Design review of the part built by this model. Coordinates are the model's own, in mm. A direction names the side the tool comes from. Coordinates: 2 decimals unless noted, no trailing zeros. Loops run counter-clockwise (first coordinate to the right, second up) from the corner with the lowest first, then second, coordinate; pieces in that order, holes last. Notation, with made-up numbers: M -39.75,-20 L 11.25,-20 A28 ccw 11.25,8 Z; hole C -21,-18 d10. An arc over 180 degrees is marked long. Answer as CSV lines item,"result". Start each with the question number.
from build123d import *

# Parameters (mm, degrees)
PAD002_DEPTH    = 7
SKETCH025_R     = 3
POCKET018_DEPTH = 15
POCKET019_DEPTH = 98.908358
SKETCH028_R     = 3
POCKET021_DEPTH = 7.001


with BuildPart() as part:
    # Sketch023 → Pad002 (new body)
    with BuildSketch(Plane.XY):
        with BuildLine():
            Line((75.261973, 88.907358), (50.261973, 88.907358))
            Line((50.261973, 84.907358), (50.261973, 88.907358))
            Line((50.261973, 84.907358), (20.261973, 84.907358))
            Line((-9.396926, 3.420201), (20.261973, 84.907358))
            ThreePointArc((-9.396926, 3.420201), (-4.942745, -8.693059), (7.744606, -6.326221))
            Line((7.744606, -6.326221), (52.028155, 47.886022))
            ThreePointArc((75.261973, 58.907358), (62.404289, 56.012339), (52.028155, 47.886022))
            Line((75.261973, 88.907358), (75.261973, 58.907358))
        make_face()
    extrude(amount=PAD002_DEPTH)

    # Sketch025 (on Face4 of Pad002) → Pocket018 (cut)
    with BuildSketch(Plane(origin=(0, 84.907358, 0), x_dir=(-1, 0, 0), z_dir=(0, 1, 0))):
        with Locations((-35.261973, 3.5)):
            Circle(SKETCH025_R)
    extrude(amount=-POCKET018_DEPTH, mode=Mode.SUBTRACT)

    # Sketch026 (on Face2 of Pocket018) → Pocket019 (cut, through all)
    with BuildSketch(Plane(origin=(0, 88.907358, 0), x_dir=(-1, 0, 0), z_dir=(0, 1, 0))):
        Polygon((-75.261973, 7), (-75.261973, 0), (-71.220521, 7), align=None)
    extrude(amount=-POCKET019_DEPTH, mode=Mode.SUBTRACT)

    # Sketch028 → Pocket021 (cut, through all)
    with BuildSketch(Plane.XY.offset(7)):
        with Locations((54.303425, 73.770624)):
            Circle(SKETCH028_R)
    extrude(amount=-POCKET021_DEPTH, mode=Mode.SUBTRACT)


with BuildPart() as part_1:
    # Body002 placement: moved
    add(part.part.moved(Location((-250, 0, 0))))


with BuildPart() as part_2:
    # Clone placement: moved
    add(part_1.part.moved(Location((262, 76, 0))))


solid = part_2.part
Item 1: Mouldability with a two-part tool opening along Z and no side actions: class faces 1 (the face through (50.26, 153.51, 3.63)), 2 (the face through (47.5, 160.907, 0.3)), 3 (the face through (85.27, 149.98, 3.45)) as released by +Z, released by -Z, zero draft, split by the parting line, or undercut.
Item 2: For pin 1 (2 mm diameter, centred on x = 40.5, z = 4, fed in from +Y); pin 2 (1.5 mm diameter, centred on x = 21, z = 2, fed in from -Y); pin 3 (1.8 mm diameter, centred on x = 46, z = 5, fed in from +Y), all flat-tipped, find the tip position at first contact; note any pin that passes through.
Item 3: Add section C-C (y = 99). Give the boundary of the cut face in (x, z).
Item 4: Add section A-A (z = 3.5). Give the boundary of the cut face in (x, y).
Item 5: For faces 4 (the face through (62.262, 163, 3)), 5 (the face through (47, 145.907, 4)), 6 (the face through (65.913, 152.745, 3.549)), list the 3-axis set-ups (+Z, -Z, +X, -X, +Y, -Y) from which the entire face can be reached by the end or side of a thin tool; tool diameter is ignored.
Item 6: For line 1 along Y through (x, z) = (69, 2); line 2 along X through (y, z) = (110, 5.25); line 3 along Y through (x, z) = (34.5, 1), list the stretches that pass through material, from the lowest coordinate up. Write a range as from..to.
Item 7: Add section B-B (x = 13.5). Give the boundary of the cut face in (y, z), plus the area to 3 significant figures.
Response:
1,face 1,"undercut"
1,face 2,"zero draft"
1,face 3,"released by +Z"
2,pin 1,"y = 160.91"
2,pin 2,"y = 70.29"
2,pin 3,"y = 145.91"
3,outline,"M 9.73,0 L 43.7,0 L 43.7,7 L 9.73,7 Z"
4,outline,"M 2.6,79.42 A10 ccw 19.74,69.67 L 64.03,123.89 A30 cw 85.24,134.84 L 85.24,164.91 L 62.26,164.91 L 62.26,160.91 L 50.26,160.91 L 50.26,145.91 L 44.26,145.91 L 44.26,160.91 L 32.26,160.91 Z; hole C 66.3,149.77 d6"
5,face 4,"+Z, -Z, -X, +Y"
5,face 5,"+Y"
5,face 6,"+Z, -Z"
6,line 1,"128.71..148.46, 151.09..164.91"
6,line 2,"13.73..52.69"
6,line 3,"87.74..160.91"
7,outline,"M 66.11,0 L 109.36,0 L 109.36,7 L 66.11,7 Z"
7,area,"303 mm²"
